For this review, take the finished solid that the model builds, in its own axes (mm). Face numbers are marked on the shaded views. A direction names the side the tool comes from. Give positions to 0.01 mm unless a question says otherwise; leave off trailing zeros. Write each loop counter-clockwise with the first axis right and the second up, starting at its lowest first coordinate (ties: lowest second). Pieces come first, ordered by that corner, then holes. Notation, with made-up numbers: M -22,38.5 L -2,38.5 A3 ccw -2,42.5 Z; hole C 74,-31 d9. An arc over 180 degrees is marked long. One line per item, written item: value. Start each with the question number.
Item 1: Consider section C-C, the plane y = -10.5. Write out the cut boundary in (x, z).
Item 2: Clearance check with flat-ended pins moving along their axes: pin 1 Ø10 at (x, z) = (19.5, -7) entering from +Y; pin 2 Ø4.5 at (x, z) = (-37, 22) entering from -Y; pin 3 Ø1.9 at (x, z) = (-37, -22) entering from -Y; pin 4 Ø3 at (x, z) = (-37, -22) entering from -Y. State where each tip first meets the part, or that it passes through.
Item 3: Mouldability with a two-part tool opening along X and no side actions: class the marked faces 6, 7 and 8 as released by +X, released by -X, zero draft, split by the parting line, or undercut.
Item 4: Tool access review of the marked faces 1, 2, 3, 4 and 5: name each direction out of +Z, -Z, +X, -X, +Y, -Y from which nothing blocks a thin tool from reaching the whole face with its end or side.
Item 5: To check wall thickness, follow probe 1 along X at (y, z) = (-23.75, -22) (3 decimals); probe 2 along Z at (x, y) = (37, -23.25) (3 decimals); probe 3 along Z at (x, y) = (37, -2.75). State the ranges of each line that lie inside material, in increasing order.
Item 6: Consider section A-A, the plane y = -26.25. Write out the cut boundary in (x, z) (3 decimals), and give its area (3 significant figures).
Item 7: Consider section D-D, the plane z = 18. Write out the cut boundary in (x, y), and give its area (3 significant figures).
Item 8: Consider section B-B, the plane x = -19.5. Write out the cut boundary in (y, z), and give its area (3 significant figures).
Autodesk Inventor part; units mm, degrees
ref_plane "YZ Plane" through (0, 0, 0) normal (1, 0, 0) x (0, 1, 0)
ref_plane "XZ Plane" through (0, 0, 0) normal (0, 1, 0) x (-1, 0, 0)
ref_plane "XY Plane" through (0, 0, 0) normal (0, 0, 1) x (1, 0, 0)
sketch "Sketch1" plane through (0, 0, 0) normal (0, 1, 0) x (-1, 0, 0)
  line L0 (-37, 22) -> (37, 22) construction
  line L1 (37, 22) -> (37, -22) construction
  line L2 (37, -22) -> (-37, -22) construction
  line L3 (-37, -22) -> (-37, 22) construction
  line L4 (-37, 22) -> (37, -22) construction
  line L5 (37, 22) -> (-37, -22) construction
  line L6 (-47, 32) -> (47, 32) construction
  line L7 (47, 32) -> (47, -32) construction
  line L8 (47, -32) -> (-47, -32) construction
  line L9 (-47, -32) -> (-47, 32) construction
  line L10 (-47, 32) -> (47, -32) construction
  line L11 (47, 32) -> (-47, -32) construction
  line L12 (31, 16) -> (43, 16)
  line L13 (43, 16) -> (43, 28)
  line L14 (43, 28) -> (31, 28)
  line L15 (31, 28) -> (31, 16)
  line L16 (31, 16) -> (43, 28) construction
  line L17 (43, 16) -> (31, 28) construction
  line L18 (47, 0) -> (-47, 0) construction
  line L19 (0, 32) -> (0, -32) construction
  line L20 (37, -22) -> (-37, 22) construction
  line L21 (47, -32) -> (-47, 32) construction
  line L22 (31, -16) -> (43, -16)
  line L23 (43, -16) -> (43, -28)
  line L24 (43, -28) -> (31, -28)
  line L25 (31, -28) -> (31, -16)
  line L26 (31, -16) -> (43, -28) construction
  line L27 (43, -16) -> (31, -28) construction
  line L28 (-31, 16) -> (-43, 16)
  line L29 (-43, 16) -> (-43, 28)
  line L30 (-43, 28) -> (-31, 28)
  line L31 (-31, 28) -> (-31, 16)
  line L32 (-31, -16) -> (-43, -16)
  line L33 (-31, -28) -> (-31, -16)
  line L34 (-43, -28) -> (-31, -28)
  line L35 (-43, -16) -> (-43, -28)
  line L36 (43, 28) -> (-43, 28)
  line L37 (-43, 28) -> (-43, -28)
  line L38 (-43, -28) -> (43, -28)
  line L39 (43, -28) -> (43, 28)
  point P0 (0, 0)
  dimension "d0" = 74
  dimension "d1" = 44
  dimension "d2" = 10
  dimension "d3" = 10
  dimension "d4" = 12
  dimension "d5" = 12
extrude "Extrusion1" add sketch "Sketch1" against normal blind 5
extrude "Extrusion2" add sketch "Sketch1" against normal blind 30 contours L15 L14 L13 L12 | L23 L24 L25 L22 | L31 L28 L29 L30 | L34 L35 L32 L33
hole "Hole2" at (-37, 0, 22) at (-37, 0, -22) at (37, 0, -22) at (37, 0, 22) direction (0, -1, 0) diameter 2.4 depth 8 tip angle 118
sketch "Sketch4" plane through (0, -30, 0) normal (0, -1, 0) x (1, 0, 0)
  line L0 (31, 28) -> (-31, 28)
  line L1 (-43, 16) -> (-31, 16)
  line L2 (31, 28) -> (-31, 28)
  line L3 (-31, 28) -> (-31, 16)
  line L4 (-31, 16) -> (31, 16)
  line L5 (31, 16) -> (31, 28)
  line L6 (43, -28) -> (-43, -28)
  line L7 (-43, -16) -> (-31, -16)
  line L8 (31, -28) -> (-31, -28)
  line L9 (-31, -28) -> (-31, -16)
  line L10 (-31, -16) -> (31, -16)
  line L11 (31, -16) -> (31, -28)
  point P0 (0, 0)
extrude "Extrusion3" add sketch "Sketch4" against normal blind 10
sketch "Sketch5" plane through (0, -30, 0) normal (0, -1, 0) x (1, 0, 0)
  circle A0 centre (37, 22) radius 1.2
  circle A1 centre (-37, 22) radius 1.2
  circle A2 centre (-37, -22) radius 1.2
  circle A3 centre (37, -22) radius 1.2
  point P0 (0, 0)
hole "Hole3" at (37, -30, 22) at (-37, -30, 22) at (-37, -30, -22) at (37, -30, -22) direction (0, 1, 0) diameter 5.35 depth 10 tip angle 118
properties part number "PCB_Housing_01"
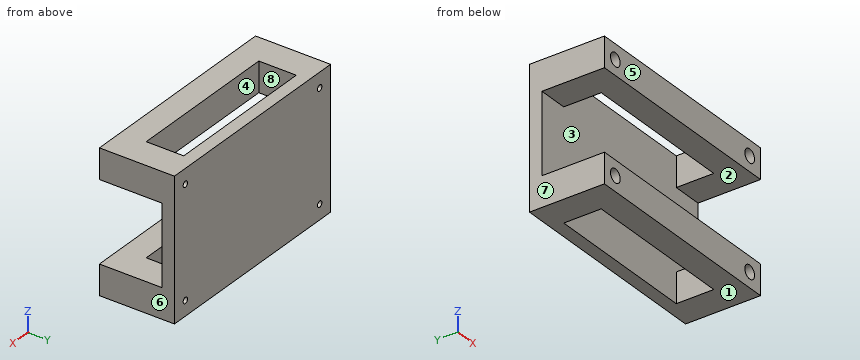
Model answer:
1. outline: M -43,-28 L -31,-28 L -31,-16 L -43,-16 Z; M -43,16 L -31,16 L -31,28 L -43,28 Z; M 31,-28 L 43,-28 L 43,-16 L 31,-16 Z; M 31,16 L 43,16 L 43,28 L 31,28 Z
2. pin 1: stops at y = 0
2. pin 2: stops at y = -19.74
2. pin 3: stops at y = -18.96
2. pin 4: stops at y = -19.29
3. face 6: released by +X
3. face 7: released by -X
3. face 8: undercut
4. face 1: -Z, +X, -X, +Y, -Y
4. face 2: +X, -X, -Y
4. face 3: none
4. face 4: +Z, -Z
4. face 5: +Z, -Z, +X, -X, -Y
5. probe 1: x = -43 to -39.675, -34.325 to 34.325, 39.675 to 43
5. probe 2: z = -28 to -24.675, -19.325 to -16, 16 to 19.325, 24.675 to 28
5. probe 3: z = -28 to -23.2, -20.8 to 20.8, 23.2 to 28
6. outline: M -43,-28 L 43,-28 L 43,-16 L -43,-16 Z; M -43,16 L 43,16 L 43,28 L -43,28 Z; hole C -37,-22 d5.35; hole C -37,22 d5.35; hole C 37,-22 d5.35; hole C 37,22 d5.35
6. area: 1,970 mm2
7. outline: M -43,-30 L 43,-30 L 43,0 L -43,0 Z; hole M -31,-20 L 31,-20 L 31,-5 L -31,-5 Z
7. area: 1,650 mm2
8. outline: M -30,-28 L -20,-28 L -20,-16 L -30,-16 Z; M -30,16 L -20,16 L -20,28 L -30,28 Z; M -5,-28 L 0,-28 L 0,28 L -5,28 Z
8. area: 520 mm2
